The drawing under review shows one solid part. Ordinate dimensions are in mm from its lowest x, y, z. A direction names the side the tool comes from. Coordinates: 2 decimals unless noted, no trailing zeros. Order: outer loops, then holes, each group sorted by start corner. A loop starts at its lowest first (then second) coordinate and runs counter-clockwise, first axis right, second up. Notation, with made-up numbers: (1.25, 82) - (13.25, 82) arc R22 cw to (13.25, 119) - close; hole circle Ø3 at (-9, 74). An arc over 180 degrees is marked (long way). Write item = value, one per line. Start each with the question number.
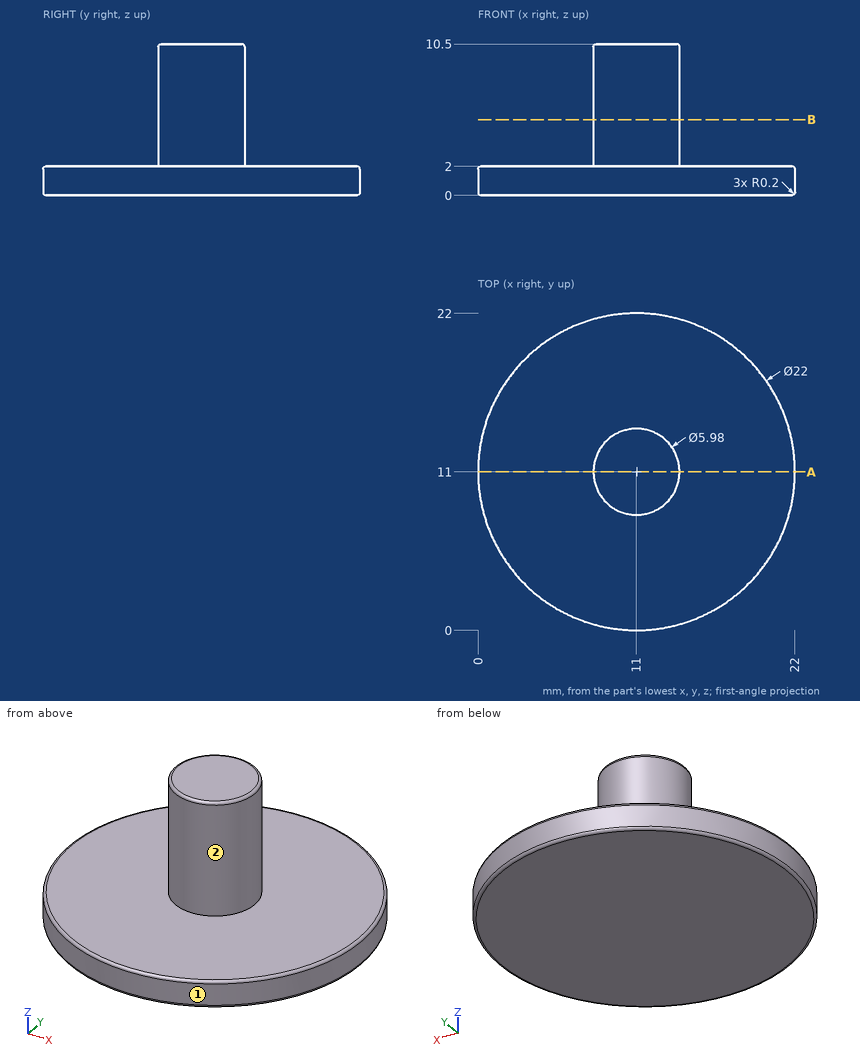
Item 1: For P1, Ø4, axis at y = 13, z = 8, coming from the +X side; P2, Ø5, axis at y = 7.5, z = 3, coming from the -X side; P3, Ø6, axis at x = 13, z = 6.5, coming from the +Y side, all flat-tipped, find the tip position at first contact; note any pin that passes through.
Item 2: Add section A-A on y = 11. Give the boundary of the cut face in (x, z), plus the area to 3 significant figures.
Item 3: Add section B-B on z = 5.25. Give the boundary of the cut face in (x, y), plus the area to 3 significant figures.
Item 4: For line 1 (Z direction, x = 19, y = 10.5); line 2 (X direction, y = 10.5, z = 2.75); line 3 (X direction, y = 3, z = 0.5), list the stretches that pass through material, from the lowest coordinate up.
Item 5: For the marked faces 1 and 2, list the 3-axis set-ups (+Z, -Z, +X, -X, +Y, -Y) from which the entire face can be reached by the end or side of a thin tool; tool diameter is ignored.
Worked out:
q1.P1 = 13.99
q1.P2 = 0.08
q1.P3 = 13.99
q2.outline = (0, 0.2) arc R0.2 ccw to (0.2, 0) - (21.8, 0) arc R0.2 ccw to (22, 0.2) - (22, 1.8) arc R0.2 ccw to (21.8, 2) - (13.99, 2) - (13.99, 10.3) arc R0.2 ccw to (13.79, 10.5) - (8.21, 10.5) arc R0.2 ccw to (8.01, 10.3) - (8.01, 2) - (0.2, 2) arc R0.2 ccw to (0, 1.8) - close
q2.area = 94.8 mm2
q3.outline = circle Ø5.98 at (11, 11)
q3.area = 28.1 mm2
q4.line_1 = 0 to 2
q4.line_2 = 8.05 to 13.95
q4.line_3 = 3.45 to 18.55
q5.face_1 = +Z, -Z
q5.face_2 = +Z
